Source: CAD feature listing. Evaluate the final solid. Frame: model axes, mm. Face numbers are marked on the shaded views. A direction names the side the tool comes from. Coordinates: 2 decimals unless noted, no trailing zeros. Loops run counter-clockwise (first coordinate to the right, second up) from the corner with the lowest first, then second, coordinate; pieces in that order, holes last.
Item 1: Reachability of the marked faces 1 and 2 from +Z, -Z, +X, -X, +Y, -Y: full face, straight path, thin tool, end or side. Return the list, or none.
Item 2: Line query: probe 1 along Y at (x, z) = (-343, 125); probe 2 along X at (y, z) = (27.5, -60); probe 3 along Y at (x, z) = (0, -145.25). Output: solid intervals per line, ascending.
Item 3: Section query A-A, the plane x = 0. Return the cut outline in (y, z), then the cut area to 3 significant figures.
Item 4: Pin query (flat end, axial travel): pin 1 Ø1 at (x, y) = (18.5, 107) entering from -Z; pin 2 Ø8 at (x, z) = (-255, 2.5) entering from +Y. Return the tip coordinate at first contact, or that it passes through.
Item 5: Pull-direction query (Z, two-part tool) for the marked faces 3, 4, 5 and 6; classes: +Z half, -Z half, draft (parallel to the pull), parting line (faces both ways), or undercut.
Item 6: Section query B-B, the plane x = -244. Return the cut outline in (y, z).
Item 7: Section query D-D, the plane y = 92. Return the cut outline in (x, z).
Item 8: Section query C-C, the plane z = -19. Return the cut outline in (x, y).
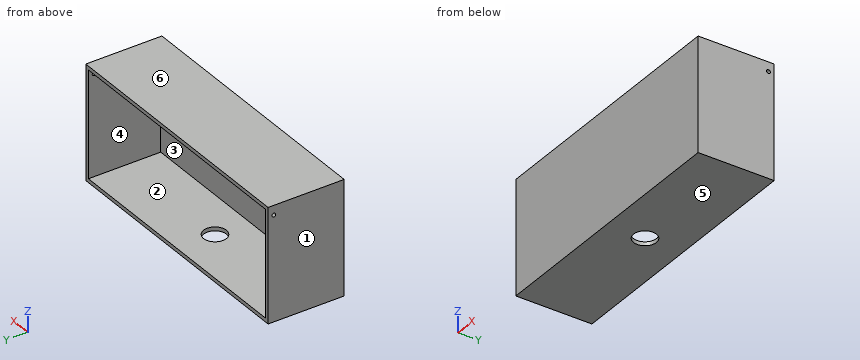
```python
from build123d import *

# Parameters (mm, degrees)
CROQUIS1_W              = 700
CROQUIS1_H              = 300
SALIENTE_EXTRUIR1_DEPTH = 200
CROQUIS2_W              = 680
CROQUIS2_H              = 280
CORTAR_EXTRUIR1_DEPTH   = 190
CROQUIS3_R              = 5
CORTAR_EXTRUIR2_DEPTH   = 700
CROQUIS4_R              = 30
CORTAR_EXTRUIR3_DEPTH   = 10


with BuildPart() as part:
    # Croquis1 → Saliente-Extruir1 (new body)
    with BuildSketch(Plane(origin=(0, 0, 0), x_dir=(1, 0, 0), z_dir=(0, 1, 0))):
        Rectangle(CROQUIS1_W, CROQUIS1_H)
    extrude(amount=SALIENTE_EXTRUIR1_DEPTH)

    # Croquis2 → Cortar-Extruir1 (cut)
    with BuildSketch(Plane(origin=(0, 200, 0), x_dir=(1, 0, 0), z_dir=(0, 1, 0))):
        Rectangle(CROQUIS2_W, CROQUIS2_H)
    extrude(amount=-CORTAR_EXTRUIR1_DEPTH, mode=Mode.SUBTRACT)

    # Croquis3 → Cortar-Extruir2 (cut)
    with BuildSketch(Plane(origin=(350, 0, 0), x_dir=(0, 0, -1), z_dir=(1, 0, 0))):
        with Locations((-125, 185)):
            Circle(CROQUIS3_R)
    extrude(amount=-CORTAR_EXTRUIR2_DEPTH, mode=Mode.SUBTRACT)

    # Croquis4 → Cortar-Extruir3 (cut)
    with BuildSketch(Plane(origin=(0, 0, -150), x_dir=(-1, 0, 0), z_dir=(0, 0, -1))):
        with Locations((0, 100)):
            Circle(CROQUIS4_R)
    extrude(amount=-CORTAR_EXTRUIR3_DEPTH, mode=Mode.SUBTRACT)


solid = part.part
```
Verdict:
1. face 1: +Z, -Z, -X, +Y, -Y
1. face 2: +Y
2. probe 1: y = 0 to 180, 190 to 200
2. probe 2: x = -350 to -340, 340 to 350
2. probe 3: y = 0 to 70, 130 to 200
3. outline: (0, -150) - (70, -150) - (70, -140) - (10, -140) - (10, 140) - (200, 140) - (200, 150) - (0, 150) - close; (130, -150) - (200, -150) - (200, -140) - (130, -140) - close
3. area: 6,200 mm2
4. pin 1: stops at z = 140
4. pin 2: stops at y = 10
5. face 3: undercut
5. face 4: undercut
5. face 5: -Z half
5. face 6: +Z half
6. outline: (0, -150) - (200, -150) - (200, -140) - (10, -140) - (10, 140) - (200, 140) - (200, 150) - (0, 150) - close
7. outline: (-350, -150) - (-28.91, -150) - (-28.91, -140) - (-340, -140) - (-340, 140) - (340, 140) - (340, -140) - (28.91, -140) - (28.91, -150) - (350, -150) - (350, 150) - (-350, 150) - close
8. outline: (-350, 0) - (350, 0) - (350, 200) - (340, 200) - (340, 10) - (-340, 10) - (-340, 200) - (-350, 200) - close
